The listing builds one solid part. Answer for the finished solid, in the listing's coordinates (mm). Round coordinates to 2 decimals unless told otherwise and drop trailing zeros. Order: outer loops, then holes, each group sorted by start corner. A loop starts at its lowest first (then second) coordinate and runs counter-clockwise, first axis right, second up. Notation, with made-up numbers: M 67.5,77 L 111.5,77 A12 ccw 111.5,97 Z; hole C 78.5,-24 d9. An arc over 180 degrees is marked long. Put each result on its own line as item: value. Start each with the question number.
1. The part is cut by section A-A (y = 31.25). Give the vertices of the cut face in (x, z).
2. The part is cut by section B-B (x = 122.55). Give the vertices of the cut face in (y, z).
3. Consider line 1 (Z direction, x = 121.8, y = 21.75); line 2 (Z direction, x = 121.4, y = 39.5); line 3 (Y direction, x = 122.2, z = 106.5). Determine where each line is inside the solid, lowest interval first.
4. Each of these flat-tipped pins is pushed along its axis until it touches: pin 1 Ø1 at (x, y) = (122, 20) entering from +Z; pin 2 Ø0.5 at (x, y) = (121.5, 34) entering from -Z; pin 3 Ø0.8 at (x, y) = (121.5, 30.5) entering from +Z; pin 4 Ø8 at (y, z) = (35.5, 84) entering from -X. Where does it stop, or does it pass through?
from build123d import *

# Parameters (mm, degrees)
BOX047_W          = 5
BOX047_H          = 24
BOX047_DEPTH      = 40
BOX047_ROLL_ANGLE = -2.2
BOX046_W          = 5
BOX046_H          = 23
BOX046_DEPTH      = 36
FILLET050_R       = 2.5
BOX045_W          = 5
BOX045_H          = 24
BOX045_DEPTH      = 40
BOX045_ROLL_ANGLE = -2.2
BOX044_W          = 2
BOX044_H          = 25
BOX044_DEPTH      = 38
FILLET049_R       = 3
BOX043_W          = 5
BOX043_H          = 24
BOX043_DEPTH      = 42
BOX043_ROLL_ANGLE = -2.2
BOX042_W          = 1
BOX042_H          = 27
BOX042_DEPTH      = 40
FILLET048_R       = 4
FILLET051_R       = 1
FILLET052_R       = 0.8


with BuildPart() as cube473:
    # Box047 → Box047 (new body)
    with BuildSketch(Plane.XY):
        with Locations((2.5, 12)):
            Rectangle(BOX047_W, BOX047_H)
    extrude(amount=BOX047_DEPTH)


with BuildPart() as cube473_1:
    # Box047 roll: moved
    add(cube473.part.rotate(Axis((0, 0, 0), (1, 0, 0)), BOX047_ROLL_ANGLE))


with BuildPart() as cube473_2:
    # Box047 placement: moved
    add(cube473_1.part.moved(Location((175, -24, -1))))


with BuildPart() as fillet050:
    # Box046 → Box046 (new body)
    with BuildSketch(Plane(origin=(175, 0, 0), x_dir=(1, 0, 0), z_dir=(0, 0, 1))):
        with Locations((2.5, 11.5)):
            Rectangle(BOX046_W, BOX046_H)
    extrude(amount=BOX046_DEPTH)

    # Cut034: cut Cube473
    add(cube473_2.part, mode=Mode.SUBTRACT)


with BuildPart() as fillet050_1:
    # Cut034 placement: moved
    add(fillet050.part.moved(Location((-57, 17, 74))))

    # Fillet050
    fillet050_edges = [fillet050_1.edges().sort_by_distance(p)[0] for p in [
        (120.5, 40, 110),
        (120.5, 18.4391, 110),
        (120.5, 40, 74),
        (120.5, 17.056119, 74),
    ]]
    fillet(fillet050_edges, radius=FILLET050_R)


with BuildPart() as fillet050_2:
    # Fillet050 placement: moved
    add(fillet050_1.part.moved(Location((0, 1, 1))))


with BuildPart() as cube471:
    # Box045 → Box045 (new body)
    with BuildSketch(Plane.XY):
        with Locations((2.5, 12)):
            Rectangle(BOX045_W, BOX045_H)
    extrude(amount=BOX045_DEPTH)


with BuildPart() as cube471_1:
    # Box045 roll: moved
    add(cube471.part.rotate(Axis((0, 0, 0), (1, 0, 0)), BOX045_ROLL_ANGLE))


with BuildPart() as cube471_2:
    # Box045 placement: moved
    add(cube471_1.part.moved(Location((175, -24, -1))))


with BuildPart() as fillet049:
    # Box044 → Box044 (new body)
    with BuildSketch(Plane(origin=(175, 0, 0), x_dir=(1, 0, 0), z_dir=(0, 0, 1))):
        with Locations((1, 12.5)):
            Rectangle(BOX044_W, BOX044_H)
    extrude(amount=BOX044_DEPTH)

    # Cut033: cut Cube471
    add(cube471_2.part, mode=Mode.SUBTRACT)


with BuildPart() as fillet049_1:
    # Cut033 placement: moved
    add(fillet049.part.moved(Location((-57, 17, 74))))

    # Fillet049
    fillet049_edges = [fillet049_1.edges().sort_by_distance(p)[0] for p in [
        (119, 42, 112),
        (119, 18.515932, 112),
        (119, 42, 74),
        (119, 17.056119, 74),
    ]]
    fillet(fillet049_edges, radius=FILLET049_R)


with BuildPart() as fillet049_2:
    # Fillet049 placement: moved
    add(fillet049_1.part.moved(Location((3, 0, 0))))


with BuildPart() as cube469:
    # Box043 → Box043 (new body)
    with BuildSketch(Plane.XY):
        with Locations((2.5, 12)):
            Rectangle(BOX043_W, BOX043_H)
    extrude(amount=BOX043_DEPTH)


with BuildPart() as cube469_1:
    # Box043 roll: moved
    add(cube469.part.rotate(Axis((0, 0, 0), (1, 0, 0)), BOX043_ROLL_ANGLE))


with BuildPart() as cube469_2:
    # Box043 placement: moved
    add(cube469_1.part.moved(Location((175, -24, -1))))


with BuildPart() as fillet052:
    # Box042 → Box042 (new body)
    with BuildSketch(Plane(origin=(175, 0, 0), x_dir=(1, 0, 0), z_dir=(0, 0, 1))):
        with Locations((0.5, 13.5)):
            Rectangle(BOX042_W, BOX042_H)
    extrude(amount=BOX042_DEPTH)

    # Cut032: cut Cube469
    add(cube469_2.part, mode=Mode.SUBTRACT)


with BuildPart() as fillet052_1:
    # Cut032 placement: moved
    add(fillet052.part.moved(Location((-57, 16, 73))))

    # Fillet048
    fillet048_edges = [fillet052_1.edges().sort_by_distance(p)[0] for p in [
        (118.5, 43, 113),
        (118.5, 17.592764, 113),
        (118.5, 43, 73),
        (118.5, 16.056119, 73),
    ]]
    fillet(fillet048_edges, radius=FILLET048_R)


with BuildPart() as fillet052_2:
    # Fillet048 placement: moved
    add(fillet052_1.part.moved(Location((4, 0, 0))))

    # Fusion005: union Fillet049
    add(fillet049_2.part)

    # Cut035: cut Fillet050
    add(fillet050_2.part, mode=Mode.SUBTRACT)

    # Fillet051
    fillet051_edges = [fillet052_2.edges().sort_by_distance(p)[0] for p in [
        (123, 41, 93),
        (123, 18.751296, 93.09597),
    ]]
    fillet(fillet051_edges, radius=FILLET051_R)

    # Fillet052
    fillet052_edges = [fillet052_2.edges().sort_by_distance(p)[0] for p in [
        (123, 16.830341, 93.153551),
        (123, 43, 93),
    ]]
    fillet(fillet052_edges, radius=FILLET052_R)


solid = fillet052_2.part
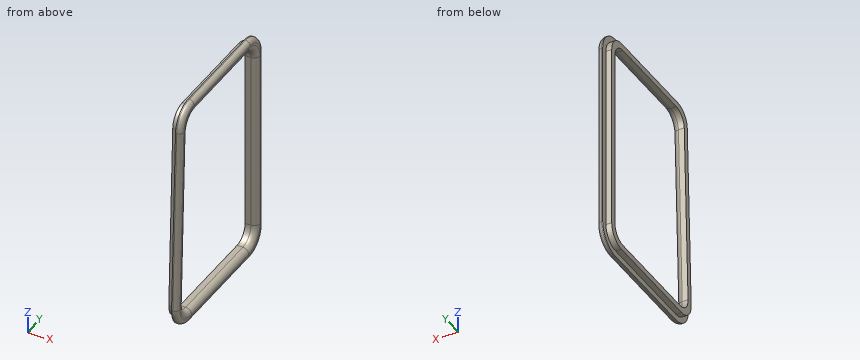
Resolved:
1. outline: M 121,74 L 122,74 L 122,73 L 122.2,73 A0.8 ccw 123,73.8 L 123,74 A1 ccw 122,75 L 121,75 Z; M 121,111 L 122,111 A1 ccw 123,112 L 123,112.2 A0.8 ccw 122.2,113 L 122,113 L 122,112 L 121,112 Z
2. outline: M 16.3,77.15 A3.92 ccw 20.21,73.08 L 39,73.08 A3.92 ccw 42.92,77 L 42.92,109 A3.92 ccw 39,112.92 L 21.44,112.92 A3.92 ccw 17.53,109.15 Z; hole M 17.99,77.6 A2.66 ccw 20.65,74.84 L 38.5,74.84 A2.66 ccw 41.16,77.5 L 41.16,108.5 A2.66 ccw 38.5,111.16 L 21.84,111.16 A2.66 ccw 19.18,108.6 Z
3. line 1: 74 to 75, 111 to 112
3. line 2: 74.04 to 75.21, 110.79 to 111.96
3. line 3: 17.34 to 19.25, 41.02 to 43
4. pin 1: z = 112.89
4. pin 2: z = 74
4. pin 3: z = 112
4. pin 4: through
